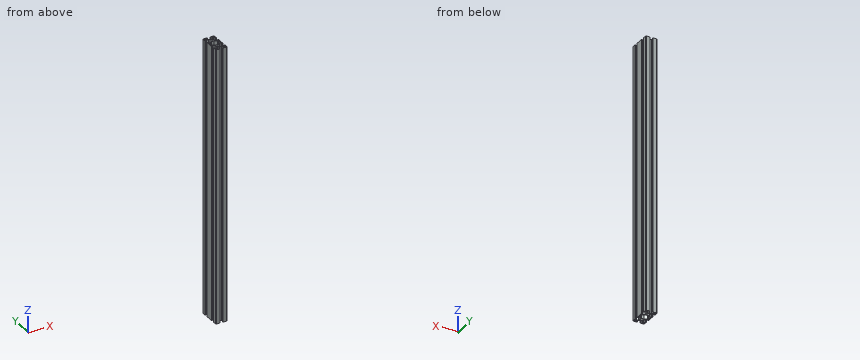
```python
from build123d import *

# Parameters (mm, degrees)
SKETCH2_R           = 2.1
SKETCH2_R_2         = 3.4
BOSS_EXTRUDE1_DEPTH = 720


with BuildPart() as part:
    # Sketch2 → Boss-Extrude1 (new body)
    with BuildSketch(Plane.XY):
        with BuildLine():
            Line((-13, -30), (-4.3, -30))
            ThreePointArc((-4.3, -30), (-4.087867966, -29.912132034), (-4, -29.7))
            Line((-4, -29.7), (-4, -28))
            Line((-4, -28), (-8.249999995, -28))
            Line((-8.249999995, -28), (-8.249999995, -24.664213567))
            Line((-8.249999995, -24.664213567), (-4.585786428, -21))
            Line((-4.585786428, -21), (-0.519615237, -21))
            Line((-0.519615237, -21), (5e-09, -20.7))
            Line((5e-09, -20.7), (0.519615247, -21))
            Line((0.519615247, -21), (4.585786438, -21))
            Line((4.585786438, -21), (8.250000005, -24.664213567))
            Line((8.250000005, -24.664213567), (8.250000005, -28))
            Line((8.250000005, -28), (4, -28))
            Line((4, -28), (4, -29.7))
            ThreePointArc((4, -29.7), (4.087867966, -29.912132034), (4.3, -30))
            Line((4.3, -30), (13, -30))
            ThreePointArc((13, -30), (14.414213562, -29.414213562), (15, -28))
            Line((15, -28), (15, -19.3000023))
            ThreePointArc((15, -19.3000023), (14.912132034, -19.087870266), (14.7, -19.0000023))
            Line((14.7, -19.0000023), (13.000000005, -19.0000023))
            Line((13.000000005, -19.0000023), (13.000000005, -23.250000005))
            Line((13.000000005, -23.250000005), (9.664213567, -23.250000005))
            Line((9.664213567, -23.250000005), (6.000000005, -19.585786443))
            Line((6.000000005, -19.585786443), (6.000000005, -15.519615247))
            Line((6.000000005, -15.519615247), (5.700000005, -15.000000005))
            Line((5.700000005, -15.000000005), (6.000000005, -14.480384763))
            Line((6.000000005, -14.480384763), (6.000000005, -10.414213567))
            Line((6.000000005, -10.414213567), (9.664213567, -6.750000005))
            Line((9.664213567, -6.750000005), (13.000000005, -6.750000005))
            Line((13.000000005, -6.750000005), (13.000000005, -11.0000023))
            Line((13.000000005, -11.0000023), (14.7, -11.0000023))
            ThreePointArc((14.7, -11.0000023), (14.912132034, -10.912134335), (15, -10.7000023))
            Line((15, -10.7000023), (15, 10.7000023))
            ThreePointArc((15, 10.7000023), (14.912132034, 10.912134335), (14.7, 11.0000023))
            Line((14.7, 11.0000023), (13.000000005, 11.0000023))
            Line((13.000000005, 11.0000023), (13.000000005, 6.749999995))
            Line((13.000000005, 6.749999995), (9.664213567, 6.749999995))
            Line((9.664213567, 6.749999995), (6.000000005, 10.414213557))
            Line((6.000000005, 10.414213557), (6.000000005, 14.480384753))
            Line((6.000000005, 14.480384753), (5.700000005, 14.999999995))
            Line((5.700000005, 14.999999995), (6.000000005, 15.519615237))
            Line((6.000000005, 15.519615237), (6.000000005, 19.585786433))
            Line((6.000000005, 19.585786433), (9.664213567, 23.249999995))
            Line((9.664213567, 23.249999995), (13.000000005, 23.249999995))
            Line((13.000000005, 23.249999995), (13.000000005, 19.0000023))
            Line((13.000000005, 19.0000023), (14.7, 19.0000023))
            ThreePointArc((14.7, 19.0000023), (14.912132034, 19.087870266), (15, 19.3000023))
            Line((15, 19.3000023), (15, 28))
            ThreePointArc((15, 28), (14.414213562, 29.414213562), (13, 30))
            Line((13, 30), (4.3, 30))
            ThreePointArc((4.3, 30), (4.087867966, 29.912132034), (4, 29.7))
            Line((4, 29.7), (4, 28))
            Line((4, 28), (8.250000005, 28))
            Line((8.250000005, 28), (8.250000005, 24.664213557))
            Line((8.250000005, 24.664213557), (4.585786448, 21))
            Line((4.585786448, 21), (0.519615247, 21))
            Line((0.519615247, 21), (5e-09, 20.7))
            Line((5e-09, 20.7), (-0.519615237, 21))
            Line((-0.519615237, 21), (-4.585786438, 21))
            Line((-4.585786438, 21), (-8.249999995, 24.664213557))
            Line((-8.249999995, 24.664213557), (-8.249999995, 28))
            Line((-8.249999995, 28), (-4, 28))
            Line((-4, 28), (-4, 29.7))
            ThreePointArc((-4, 29.7), (-4.087867966, 29.912132034), (-4.3, 30))
            Line((-4.3, 30), (-13, 30))
            ThreePointArc((-13, 30), (-14.414213562, 29.414213562), (-15, 28))
            Line((-15, 28), (-15, 19.3000023))
            ThreePointArc((-15, 19.3000023), (-14.912132034, 19.087870266), (-14.7, 19.0000023))
            Line((-14.7, 19.0000023), (-12.999999995, 19.0000023))
            Line((-12.999999995, 19.0000023), (-12.999999995, 23.249999995))
            Line((-12.999999995, 23.249999995), (-9.664213557, 23.249999995))
            Line((-9.664213557, 23.249999995), (-5.999999995, 19.585786433))
            Line((-5.999999995, 19.585786433), (-5.999999995, 15.519615237))
            Line((-5.999999995, 15.519615237), (-5.699999995, 14.999999995))
            Line((-5.699999995, 14.999999995), (-5.999999995, 14.480384753))
            Line((-5.999999995, 14.480384753), (-5.999999995, 10.414213557))
            Line((-5.999999995, 10.414213557), (-9.664213557, 6.749999995))
            Line((-9.664213557, 6.749999995), (-12.999999995, 6.749999995))
            Line((-12.999999995, 6.749999995), (-12.999999995, 11.0000023))
            Line((-12.999999995, 11.0000023), (-14.7, 11.0000023))
            ThreePointArc((-14.7, 11.0000023), (-14.912132034, 10.912134335), (-15, 10.7000023))
            Line((-15, 10.7000023), (-15, -10.7000023))
            ThreePointArc((-15, -10.7000023), (-14.912132034, -10.912134335), (-14.7, -11.0000023))
            Line((-14.7, -11.0000023), (-12.999999995, -11.0000023))
            Line((-12.999999995, -11.0000023), (-12.999999995, -6.750000005))
            Line((-12.999999995, -6.750000005), (-9.664213557, -6.750000005))
            Line((-9.664213557, -6.750000005), (-5.999999995, -10.414213567))
            Line((-5.999999995, -10.414213567), (-5.999999995, -14.480384763))
            Line((-5.999999995, -14.480384763), (-5.699999995, -15.000000005))
            Line((-5.699999995, -15.000000005), (-5.999999995, -15.519615247))
            Line((-5.999999995, -15.519615247), (-5.999999995, -19.585786443))
            Line((-5.999999995, -19.585786443), (-9.664213557, -23.250000005))
            Line((-9.664213557, -23.250000005), (-12.999999995, -23.250000005))
            Line((-12.999999995, -23.250000005), (-12.999999995, -19.0000023))
            Line((-12.999999995, -19.0000023), (-14.7, -19.0000023))
            ThreePointArc((-14.7, -19.0000023), (-14.912132034, -19.087870266), (-15, -19.3000023))
            Line((-15, -19.3000023), (-15, -28))
            ThreePointArc((-15, -28), (-14.414213562, -29.414213562), (-13, -30))
        make_face()
        with Locations(Location((11.625000005, 26.624999995, 0), (0, 0, 180))):
            Circle(SKETCH2_R, mode=Mode.SUBTRACT)
        with Locations(Location((11.625000005, -26.625000005, 0), (0, 0, 180))):
            Circle(SKETCH2_R, mode=Mode.SUBTRACT)
        with Locations(Location((4.55e-07, -15.00000049, 0), (0, 0, 180))):
            Circle(SKETCH2_R_2, mode=Mode.SUBTRACT)
        with Locations(Location((4.55e-07, 15.0000023, 0), (0, 0, 180))):
            Circle(SKETCH2_R_2, mode=Mode.SUBTRACT)
        with Locations(Location((-11.624999995, 26.624999995, 0), (0, 0, 180))):
            Circle(SKETCH2_R, mode=Mode.SUBTRACT)
        with Locations(Location((-11.624999995, -26.625000005, 0), (0, 0, 180))):
            Circle(SKETCH2_R, mode=Mode.SUBTRACT)
        with BuildLine():
            Line((-12.999999995, 3.749999995), (-12.999999995, -3.750000005))
            ThreePointArc((-12.999999995, -3.750000005), (-12.707106776, -4.457106786), (-11.999999995, -4.750000005))
            Line((-11.999999995, -4.750000005), (-8.835786433, -4.750000005))
            Line((-8.835786433, -4.750000005), (-3.651790591, -9.933995846))
            ThreePointArc((-3.651790591, -9.933995846), (-3.470778838, -10.020245326), (-3.275865231, -9.973203714))
            ThreePointArc((-3.275865231, -9.973203714), (1.45e-07, -9.000002005), (3.275865622, -9.973203376))
            ThreePointArc((3.275865622, -9.973203376), (3.470779219, -10.02024497), (3.651790956, -9.933995491))
            Line((3.651790956, -9.933995491), (8.835786443, -4.750000005))
            Line((8.835786443, -4.750000005), (12.000000005, -4.750000005))
            ThreePointArc((12.000000005, -4.750000005), (12.707106786, -4.457106786), (13.000000005, -3.750000005))
            Line((13.000000005, -3.750000005), (13.000000005, 3.749999995))
            ThreePointArc((13.000000005, 3.749999995), (12.707106786, 4.457106776), (12.000000005, 4.749999995))
            Line((12.000000005, 4.749999995), (8.835786443, 4.749999995))
            Line((8.835786443, 4.749999995), (3.6517913, 9.933995138))
            ThreePointArc((3.6517913, 9.933995138), (3.470779584, 10.020244614), (3.275866001, 9.973203046))
            ThreePointArc((3.275866001, 9.973203046), (1.45e-07, 9.000001815), (-3.27586561, 9.973203384))
            ThreePointArc((-3.27586561, 9.973203384), (-3.470779203, 10.020244971), (-3.651790935, 9.933995493))
            Line((-3.651790935, 9.933995493), (-8.835786433, 4.749999995))
            Line((-8.835786433, 4.749999995), (-11.999999995, 4.749999995))
            ThreePointArc((-11.999999995, 4.749999995), (-12.707106776, 4.457106776), (-12.999999995, 3.749999995))
        make_face(mode=Mode.SUBTRACT)
    extrude(amount=BOSS_EXTRUDE1_DEPTH)


solid = part.part
```
Work out the finished part from the listing and answer in its coordinate system (mm). Round coordinates to 2 decimals unless told otherwise and drop trailing zeros.
1) Consider probe 1 along Y at (x, z) = (11.25, 545.5); probe 2 along X at (y, z) = (7.5, 652); probe 3 along X at (y, z) = (-0.5, 174.5). Determine where each line is inside the solid, lowest interval first.
2) Flat-ended cylindrical pins translate along their axes: P1, Ø1.2, axis at x = 2, z = 397.5, coming from the -Y side; P2, Ø0.8, axis at y = -29, z = 379, coming from the -X side; P3, Ø0.5, axis at x = 13.5, z = 351, coming from the +Y side. Find the tip coordinate at first contact, or state that the pin passes through.
3) A cutting plane is placed at A-A on z = 106. Give the number of separate pieces and of enclosed holes in the cut face, and give its area (3 significant figures).
Entries:
1. probe 1: y = -30 to -28.69, -24.56 to -23.25, -6.75 to -4.75, 4.75 to 6.75, 23.25 to 24.56, 28.69 to 30
1. probe 2: x = -15 to -13, -8.91 to -6.09, 6.09 to 8.91, 13 to 15
1. probe 3: x = -15 to -13, 13 to 15
2. P1: stops at y = -21
2. P2: stops at x = -14.91
2. P3: stops at y = 29.98
3. separate pieces: 1
3. enclosed holes: 7
3. area: 591 mm2
